```python
from build123d import *

# Parameters (mm, degrees)
RESSALTO_EXTRUS_O2_DEPTH = 3
RESSALTO_EXTRUS_O3_START = 15
RESSALTO_EXTRUS_O3_DEPTH = 15
ESBO_O3_R                = 1.5
CORTE_EXTRUS_O1_DEPTH    = 51
ESBO_O4_R                = 1.4605
CORTE_EXTRUS_O2_DEPTH    = 50
ESBO_O5_W                = 28.5
ESBO_O5_H                = 11.5
ESBO_O5_W_2              = 27.5
ESBO_O5_H_2              = 10.5
CORTE_EXTRUS_O3_DEPTH    = 50


with BuildPart() as part:
    # Esboço1 → Ressalto-extrusão2 (new body)
    with BuildSketch(Plane.YZ):
        with BuildLine():
            Line((-13, 40), (13, 40))
            ThreePointArc((13, 40), (20.778174593, 36.778174593), (24, 29))
            Line((24, 29), (24, -40))
            Line((24, -40), (-24, -40))
            Line((-24, -40), (-24, 29))
            ThreePointArc((-24, 29), (-20.778174593, 36.778174593), (-13, 40))
        make_face()
    extrude(amount=RESSALTO_EXTRUS_O2_DEPTH)

    # Esboço2 → Ressalto-extrusão3 (add)
    with BuildSketch(Plane(origin=(0, 0, 0), x_dir=(0, -1, 0), z_dir=(-1, 0, 0)).offset(RESSALTO_EXTRUS_O3_START)):
        with BuildLine():
            Line((-13, 40), (13, 40))
            ThreePointArc((13, 40), (20.778174593, 36.778174593), (24, 29))
            Line((24, 29), (24, -40))
            Line((24, -40), (-24, -40))
            Line((-24, -40), (-24, 29))
            ThreePointArc((-24, 29), (-20.778174593, 36.778174593), (-13, 40))
        make_face()
        with BuildLine():
            Line((-20, -37), (20, -37))
            Line((20, -37), (20, 26))
            ThreePointArc((20, 26), (16.778174593, 33.778174593), (9, 37))
            Line((9, 37), (-9, 37))
            ThreePointArc((-9, 37), (-16.778174593, 33.778174593), (-20, 26))
            Line((-20, 26), (-20, -37))
        make_face(mode=Mode.SUBTRACT)
    extrude(amount=-RESSALTO_EXTRUS_O3_DEPTH)

    # Esboço3 → Corte-extrusão1 (cut, through all)
    with BuildSketch(Plane.YZ.offset(3)):
        with Locations(Location((0, 35, 0), (0, 0, 270))):
            Circle(ESBO_O3_R)
        with Locations(Location((16, -5, 0), (0, 0, 270))):
            Circle(ESBO_O3_R)
        with Locations(Location((-16, -5, 0), (0, 0, 270))):
            Circle(ESBO_O3_R)
    extrude(amount=-CORTE_EXTRUS_O1_DEPTH, mode=Mode.SUBTRACT)

    # Esboço4 → Corte-extrusão2 (cut, through all)
    with BuildSketch(Plane(origin=(0, 0, 0), x_dir=(0, -1, 0), z_dir=(-1, 0, 0))):
        with Locations(Location((7.948942217, 5.133929433, 0), (0, 0, 90))):
            Circle(ESBO_O4_R)
        with Locations(Location((-8.5738, -25.8659, 0), (0, 0, 90))):
            Circle(ESBO_O4_R)
    extrude(amount=-CORTE_EXTRUS_O2_DEPTH, mode=Mode.SUBTRACT)

    # Esboço5 → Corte-extrusão3 (cut, through all)
    # profile 1 of 2: a face of its own
    with BuildSketch(Plane(origin=(0, 0, 0), x_dir=(0, -1, 0), z_dir=(-1, 0, 0))):
        with Locations((0.25, 21.75)):
            Rectangle(ESBO_O5_W, ESBO_O5_H)
        with Locations((0.25, 21.75)):
            Rectangle(ESBO_O5_W_2, ESBO_O5_H_2, mode=Mode.SUBTRACT)
    # profile 2 of 2: a face of its own
    with BuildSketch(Plane(origin=(0, 0, 0), x_dir=(0, -1, 0), z_dir=(-1, 0, 0))):
        with Locations((0.25, 21.75)):
            Rectangle(ESBO_O5_W_2, ESBO_O5_H_2)
    extrude(amount=-CORTE_EXTRUS_O3_DEPTH, mode=Mode.SUBTRACT)


solid = part.part
```
Geometry check sheet. Reference: the model listing, model coordinates, mm. A direction names the side the tool comes from. Give positions to 0.01 mm unless a question says otherwise; leave off trailing zeros. Loops run counter-clockwise (first coordinate to the right, second up) from the corner with the lowest first, then second, coordinate; pieces in that order, holes last. Notation, with made-up numbers: M 1,12.5 L 56,12.5 A15 ccw 56,34.5 Z; hole C 65.5,65 d11. An arc over 180 degrees is marked long. Write item = value, one per line. Start each with the question number.
1. Thickness scan on probe 1 along Y at (x, z) = (0.6, -5); probe 2 along Y at (x, z) = (-12.75, -12); probe 3 along Z at (x, y) = (-7.5, -1.5). Record the ranges inside material, lowest first.
2. Section check B-B, the plane y = 0. Enter the section's corners in (x, z), plus the area to 4 significant figures.
3. Draft check along Z on faces 1 (the face through (-6, 24, -6)), 2 (the face through (1.479, 9.805, -25.081)), 3 (the face through (-6.126, 20.863, 36.692)). Enter one of: +Z half, -Z half, draft (parallel to the pull), parting line (faces both ways), or undercut.
4. Section check C-C, the plane x = -13.5. Enter the section's corners in (y, z), plus the area to 3 significant figures.
5. Tool access check on faces 4 (the face through (-7.605, -16.863, 33.692)), 5 (the face through (1, 0, 16)), 6 (the face through (-6.126, -20.692, 36.863)). Record the directions out of +Z, -Z, +X, -X, +Y, -Y that give a thin tool (end or side, any length) a straight path to the whole face; none if there is none.
6. Go/stop test with flat-tipped pins: P1, Ø4, axis at y = 16, z = -5, coming from the -X side; P2, Ø3.5, axis at y = 0, z = 35, coming from the +X side. Record where each tip stops, or that it passes through.
7. Section check A-A, the plane z = -5. Enter the section's corners in (x, y), plus the area to 3 significant figures.
8. Section check D-D, the plane y = 16. Enter the section's corners in (x, z), plus the area to 3 significant figures.
Values follow:
q1.probe_1 = -24 to -17.5, -14.5 to 14.5, 17.5 to 24
q1.probe_2 = -24 to -20, 20 to 24
q1.probe_3 = -40 to -37, 37 to 40
q2.outline = M -15,-40 L 3,-40 L 3,16 L 0,16 L 0,-37 L -15,-37 Z; M -15,37 L 0,37 L 0,36.5 L 3,36.5 L 3,40 L -15,40 Z; M 0,27.5 L 3,27.5 L 3,33.5 L 0,33.5 Z
q2.area = 286.5 mm^2
q3.face_1 = draft
q3.face_2 = undercut
q3.face_3 = +Z half
q4.outline = M -24,-40 L 24,-40 L 24,29 A11 ccw 13,40 L -13,40 A11 ccw -24,29 Z; hole M -20,-37 L 20,-37 L 20,26 A11 ccw 9,37 L -9,37 A11 ccw -20,26 Z
q4.area = 880 mm^2
q5.face_4 = -X
q5.face_5 = +X, -X
q5.face_6 = +Z, +X, -X, -Y
q6.P1 = 0
q6.P2 = 3
q7.outline = M -15,-24 L 3,-24 L 3,-17.5 L 0,-17.5 L 0,-20 L -15,-20 Z; M -15,20 L 0,20 L 0,17.5 L 3,17.5 L 3,24 L -15,24 Z; M 0,-14.5 L 3,-14.5 L 3,14.5 L 0,14.5 Z
q7.area = 246 mm^2
q8.outline = M -15,-40 L 3,-40 L 3,-6.5 L 0,-6.5 L 0,-37 L -15,-37 Z; M -15,34.49 L 0,34.49 L 0,-3.5 L 3,-3.5 L 3,39.58 L -15,39.58 Z
q8.area = 351 mm^2
